For this review, take the finished solid that the model builds, in its own axes (mm). Face numbers are marked on the shaded views. A direction names the side the tool comes from. Coordinates: 2 decimals unless noted, no trailing zeros. Order: outer loops, then holes, each group sorted by start corner. A loop starts at its lowest first (then second) coordinate and runs counter-clockwise, first axis right, second up.
from build123d import *

# Parameters (mm, degrees)
SKETCH1_R               = 2.1
SKETCH1_W               = 1.815
SKETCH1_H               = 1
SKETCH1_H_2             = 3
BOSS_EXTRUDE1_DEPTH     = 3
BOSS_EXTRUDE2_START     = 3
SKETCH1_8_W             = 1.815
SKETCH1_8_H             = 1
BOSS_EXTRUDE2_DEPTH     = 11.43
CUT_EXTRUDE2_DEPTH      = 29.869778286
CUT_EXTRUDE2_DEPTH_BACK = 29.869778286
SKETCH2_R               = 78.359
CHAMFER1_SIZE           = 2.54
BOSS_EXTRUDE3_DEPTH     = 1.27
FILLET1_R               = 7.62
FILLET5_R               = 10
FILLET6_R               = 4.92
SKETCH7_W               = 11.43
SKETCH7_H               = 5.433942037
CUT_EXTRUDE4_DEPTH      = 29.869778458
FILLET7_R               = 0.635


with BuildPart() as part:
    # Sketch1 → Boss-Extrude1 (new body)
    # profile 1 of 6: a face of its own
    with BuildSketch(Plane(origin=(0, 0, 0), x_dir=(1, 0, 0), z_dir=(0, 1, 0))):
        Polygon((6.985, -10.998674064), (5.715, -10.998674064), (5.715, -15.888674064), (5.715, -18.096674099), (17.255421897, -18.096674099), (17.255421897, -0.316674099), (-17.255421897, -0.316674099), (-17.255421897, -18.096674099), (-5.715, -18.096674099), (-5.715, -15.888674064), (-5.715, -10.998674064), (-6.985, -10.998674064), (-6.985, -5.728674064), (6.985, -5.728674064), align=None)
        with Locations(Location((-12.7, -12.078674064, 0), (0, 0, 270))):
            Circle(SKETCH1_R, mode=Mode.SUBTRACT)
        with Locations(Location((12.7, -12.078674064, 0), (0, 0, 270))):
            Circle(SKETCH1_R, mode=Mode.SUBTRACT)
    # profile 2 of 6: a face of its own
    with BuildSketch(Plane(origin=(0, 0, 0), x_dir=(1, 0, 0), z_dir=(0, 1, 0))):
        Polygon((5.715, -9.998674064), (5.715, -10.998674064), (6.985, -10.998674064), (6.985, -5.728674064), (-6.985, -5.728674064), (-6.985, -10.998674064), (-5.715, -10.998674064), (-5.715, -9.998674064), (-5.715, -6.998674064), (-3.9, -6.998674064), (3.9, -6.998674064), (5.715, -6.998674064), align=None)
    # profile 3 of 6: a face of its own
    with BuildSketch(Plane(origin=(0, 0, 0), x_dir=(1, 0, 0), z_dir=(0, 1, 0))):
        with Locations((-4.8075, -10.498674064)):
            Rectangle(SKETCH1_W, SKETCH1_H)
    # profile 4 of 6: a face of its own
    with BuildSketch(Plane(origin=(0, 0, 0), x_dir=(1, 0, 0), z_dir=(0, 1, 0))):
        with Locations((-4.8075, -8.498674064)):
            Rectangle(SKETCH1_W, SKETCH1_H_2)
    # profile 5 of 6: a face of its own
    with BuildSketch(Plane(origin=(0, 0, 0), x_dir=(1, 0, 0), z_dir=(0, 1, 0))):
        with Locations((4.8075, -8.498674064)):
            Rectangle(SKETCH1_W, SKETCH1_H_2)
    # profile 6 of 6: a face of its own
    with BuildSketch(Plane(origin=(0, 0, 0), x_dir=(1, 0, 0), z_dir=(0, 1, 0))):
        with Locations((4.8075, -10.498674064)):
            Rectangle(SKETCH1_W, SKETCH1_H)
    extrude(amount=BOSS_EXTRUDE1_DEPTH)

    # Sketch1<8> → Boss-Extrude2 (add)
    with BuildSketch(Plane(origin=(0, 0, 0), x_dir=(1, 0, 0), z_dir=(0, 1, 0)).offset(BOSS_EXTRUDE2_START)):
        Polygon((5.715, -9.998674064), (5.715, -10.998674064), (6.985, -10.998674064), (6.985, -5.728674064), (-6.985, -5.728674064), (-6.985, -10.998674064), (-5.715, -10.998674064), (-5.715, -9.998674064), (-5.715, -6.998674064), (-3.9, -6.998674064), (3.9, -6.998674064), (5.715, -6.998674064), align=None)
        with Locations((4.8075, -10.498674064)):
            Rectangle(SKETCH1_8_W, SKETCH1_8_H)
        with Locations((-4.8075, -10.498674064)):
            Rectangle(SKETCH1_8_W, SKETCH1_8_H)
    extrude(amount=BOSS_EXTRUDE2_DEPTH)

    # Sketch2 → Cut-Extrude2 (cut, two sides: drawn at the far end of the back side and taken through both)
    with BuildSketch(Plane.XY.offset(-CUT_EXTRUDE2_DEPTH_BACK)):
        with Locations((0, -76.858999952)):
            Circle(SKETCH2_R)
    extrude(amount=CUT_EXTRUDE2_DEPTH + CUT_EXTRUDE2_DEPTH_BACK, mode=Mode.SUBTRACT)

    # Chamfer1
    # the kernel refuses this chamfer: 2.54 mm, written as the material it adds along each edge
    with BuildSketch(Plane(origin=(5.715, 3, 6.998674064), x_dir=(0.027495876610586268, 0.9996219169112968, 0), z_dir=(0, 0, 1))) as chamfer1_piece_1_section:
        Polygon((CHAMFER1_SIZE * 0.999621916911, CHAMFER1_SIZE * 0.0274958766106), (-CHAMFER1_SIZE * 0.0274958766106, CHAMFER1_SIZE * 0.999621916911), (0, 0), align=None)
    chamfer1_piece_1 = extrude(amount=3, mode=Mode.PRIVATE)
    chamfer1_piece_1 = split(chamfer1_piece_1, bisect_by=Plane(origin=(3.9, 3.90032925, 8.498674064), z_dir=(1, 0, 0)), keep=Keep.TOP, mode=Mode.PRIVATE)
    add(chamfer1_piece_1)
    with BuildSketch(Plane(origin=(-5.715, 3, 9.998674064), x_dir=(-0.027495876610586268, 0.9996219169112968, 0), z_dir=(0, 0, -1))) as chamfer1_piece_2_section:
        Polygon((CHAMFER1_SIZE * 0.999621916911, CHAMFER1_SIZE * 0.0274958766106), (-CHAMFER1_SIZE * 0.0274958766106, CHAMFER1_SIZE * 0.999621916911), (0, 0), align=None)
    chamfer1_piece_2 = extrude(amount=3, mode=Mode.PRIVATE)
    chamfer1_piece_2 = split(chamfer1_piece_2, bisect_by=Plane(origin=(-3.9, 3.90032925, 8.498674064), z_dir=(-1, 0, 0)), keep=Keep.TOP, mode=Mode.PRIVATE)
    add(chamfer1_piece_2)

    # Sketch6 → Boss-Extrude3 (add, symmetric)
    with BuildSketch(Plane(origin=(0, 0, 0), x_dir=(0, 0, -1), z_dir=(1, 0, 0))):
        Polygon((-5.728674064, 14.43), (-0.316674099, 3), (-5.728674064, 3), align=None)
    extrude(amount=BOSS_EXTRUDE3_DEPTH, both=True)

    # Fillet1
    fillet1_edges = [part.edges().sort_by_distance(p)[0] for p in [
        (-17.255421897, 1.5, 0.316674099),
        (17.255421897, 1.5, 0.316674099),
        (17.255421897, 1.5, 18.096674099),
        (-17.255421897, 1.5, 18.096674099),
    ]]
    fillet(fillet1_edges, radius=FILLET1_R)

    # Fillet5
    # the kernel refuses this fillet: 10 mm, written as the material it adds along each edge
    with BuildSketch(Plane(origin=(-1.27, 3, 5.728674064), x_dir=(-1, 0, 0), z_dir=(0, 1, 0))) as fillet5_piece_1_section:
        with BuildLine():
            CenterArc((10, -9.03541781), FILLET5_R, 115.372403981, 64.627596019)
            Line((0, -9.03541781), (0, 0))
            Line((0, 0), (5.715, 0))
        make_face()
    fillet5_piece_1 = extrude(amount=34.018544525, mode=Mode.PRIVATE)
    fillet5_piece_1 = split(fillet5_piece_1, bisect_by=Plane(origin=(-3.934188125, 8.906839934, 3.113508527), z_dir=(0, -0.42794357624145657, 0.9038054522703837)), keep=Keep.TOP, mode=Mode.PRIVATE)
    add(fillet5_piece_1)
    with BuildSketch(Plane(origin=(1.27, 3, 5.728674064), x_dir=(1, 0, 0), z_dir=(0, 1, 0))) as fillet5_piece_2_section:
        with BuildLine():
            CenterArc((10, 9.03541781), FILLET5_R, 180, 64.627596019)
            Line((0, 9.03541781), (0, 0))
            Line((0, 0), (5.715, 0))
        make_face()
    fillet5_piece_2 = extrude(amount=34.018544525, mode=Mode.PRIVATE)
    fillet5_piece_2 = split(fillet5_piece_2, bisect_by=Plane(origin=(3.934188125, 8.906839934, 3.113508527), z_dir=(0, -0.42794357624145657, 0.9038054522703837)), keep=Keep.TOP, mode=Mode.PRIVATE)
    add(fillet5_piece_2)

    # Fillet6
    fillet6_edges = [part.edges().sort_by_distance(p)[0] for p in [
        (6.985, 8.715, 5.728674064),
        (-6.985, 8.715, 5.728674064),
    ]]
    fillet(fillet6_edges, radius=FILLET6_R)

    # Sketch7 → Cut-Extrude4 (cut, through all)
    with BuildSketch(Plane(origin=(0, 14.43, 0), x_dir=(1, 0, 0), z_dir=(0, 1, 0))):
        with Locations((0, -9.715645083)):
            Rectangle(SKETCH7_W, SKETCH7_H)
    extrude(amount=-CUT_EXTRUDE4_DEPTH, mode=Mode.SUBTRACT)

    # Fillet7
    fillet7_edges = [part.edges().sort_by_distance(p)[0] for p in [
        (6.985, 8.715, 10.998674064),
        (-6.985, 8.715, 10.998674064),
    ]]
    fillet(fillet7_edges, radius=FILLET7_R)


solid = part.part
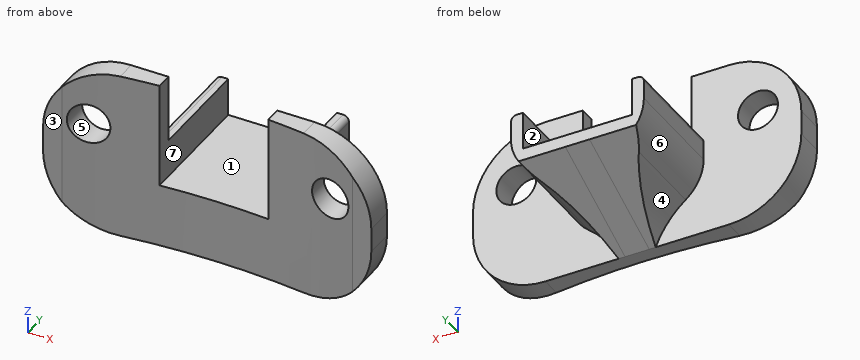
1. Take a section at B-B, the plane x = 12.7. Give the boundary of the cut face in (y, z), plus the area to 3 significant figures.
Answer below:
outline: (0.46, 0.96) - (3, 0.96) - (3, 9.98) - (0.46, 9.98) - close; (0.46, 14.18) - (3, 14.18) - (3, 17.45) - (0.46, 17.45) - close
area: 31.2 mm2
2. To check wall thickness, follow L1, parallel to X at y = 1.5, z = 9.25 (3 decimals); L2, parallel to X at y = 6.25, z = 8.5 (3 decimals); L3, parallel to Y at x = -6, z = 8. State the ranges of each line that lie inside material, in increasing order.
Answer below:
L1: x = -17.255 to -5.715, 5.715 to 17.255
L2: x = -6.985 to -5.715, 5.715 to 6.985
L3: y = 1.27 to 14.43
3. Machinability: for the marked faces 5, 6 and 7, which of the approach directions +Z, -Z, +X, -X, +Y, -Y give a long, thin tool a straight path to every point of the face, cutting with its end or side? Answer none if there is none.
Answer below:
face 5: +Y, -Y
face 6: -Z, -X, +Y
face 7: +Z, +Y, -Y
4. Take a section at D-D, the plane x = -3. Give the boundary of the cut face in (y, z).
Answer below:
outline: (1.44, 0.32) - (3, 0.32) - (3, 2.32) - (7.22, 2.32) - (14.43, 5.73) - (14.43, 7) - (1.44, 7) - close
5. Clearance check with flat-ended pins moving along their axes: pin 1 Ø4.5 at (x, z) = (12, 10) entering from +Y; pin 2 Ø2 at (x, y) = (6, 9) entering from +Z; pin 3 Ø6 at (y, z) = (10, 9) entering from +X (3 decimals). State where each tip first meets the part, or that it passes through.
Answer below:
pin 1: stops at y = 3
pin 2: stops at z = 11
pin 3: stops at x = 6.985
6. Take a section at C-C, the plane z = 7.5. Give the boundary of the cut face in (x, y) (3 decimals).
Answer below:
outline: (-17.243, 0) - (-15.259, 0) arc R78.359 cw to (-5.715, 1.291) - (-5.715, 14.43) - (-6.895, 14.43) - (-6.895, 3) - (-17.243, 3) - close; (5.715, 1.291) arc R78.359 cw to (15.259, 0) - (17.243, 0) - (17.243, 3) - (6.895, 3) - (6.895, 14.43) - (5.715, 14.43) - close
7. The part is to be moulded in two halves that separate along X. For the marked faces 1, 2, 3 and 4, say which applies: +X half, -X half, draft (parallel to the pull), parting line (faces both ways), or undercut.
Answer below:
face 1: undercut
face 2: undercut
face 3: draft
face 4: -X half
8. Take a section at A-A, the plane z = 12.25. Give the boundary of the cut face in (x, y) (3 decimals), plus the area to 3 significant figures.
Answer below:
outline: (-17.046, 0) - (-15.259, 0) arc R78.359 cw to (-14.793, 0.091) - (-14.793, 3) - (-17.046, 3) - close; (-10.607, 0.779) arc R78.359 cw to (-5.715, 1.291) - (-5.715, 3) - (-10.607, 3) - close; (5.715, 1.291) arc R78.359 cw to (10.607, 0.779) - (10.607, 3) - (5.715, 3) - close; (14.793, 0.091) arc R78.359 cw to (15.259, 0) - (17.046, 0) - (17.046, 3) - (14.793, 3) - close
area: 32.4 mm2
